from build123d import *

# Parameters (mm, degrees)
F1_DEPTH = 50
F3_D     = 3.3


with BuildPart() as f1:
    # F0 (on Front) → F1 (new body)
    with BuildSketch(Plane.XZ):
        with BuildLine():
            ThreePointArc((-2.9195071176, 0.3029216067), (-2.5916918532, 0.0788381268), (-2.2025121988, 0))
            Line((-2.2025121988, 0), (2.2025121988, 0))
            ThreePointArc((2.2025121988, 0), (2.5916918532, 0.0788381268), (2.9195071176, 0.3029216067))
            Line((2.9195071176, 0.3029216067), (5.1084974594, 2.5544545297))
            ThreePointArc((5.1084974594, 2.5544545297), (5.2132756899, 2.7149096091), (5.25, 2.9029937263))
            Line((5.25, 2.9029937263), (5.25, 3.2))
            ThreePointArc((5.25, 3.2), (5.1035533906, 3.5535533906), (4.75, 3.7))
            Line((4.75, 3.7), (3, 3.7))
            Line((3, 3.7), (3, 7))
            Line((3, 7), (-3, 7))
            Line((-3, 7), (-3, 3.7))
            Line((-3, 3.7), (-4.75, 3.7))
            ThreePointArc((-4.75, 3.7), (-5.1035533906, 3.5535533906), (-5.25, 3.2))
            Line((-5.25, 3.2), (-5.25, 2.9029937263))
            ThreePointArc((-5.25, 2.9029937263), (-5.2132756899, 2.7149096091), (-5.1084974594, 2.5544545297))
            Line((-5.1084974594, 2.5544545297), (-2.9195071176, 0.3029216067))
        make_face()
    extrude(amount=F1_DEPTH)

    # F3 (through all)
    with Locations(Plane.XY.offset(7)):
        with Locations((0, -42.5), (0, -7.5)):
            Hole(F3_D / 2)


solid = f1.part
Can you work these out from the model? Positions are in its coordinate system, mm. A direction names the side the tool comes from. Coordinates: 2 decimals unless noted, no trailing zeros. Order: outer loops, then holes, each group sorted by start corner. A loop starts at its lowest first (then second) coordinate and runs counter-clockwise, first axis right, second up. Notation, with made-up numbers: (52.25, 87) - (72.25, 87) arc R19 cw to (72.25, 123) - close; hole circle Ø9 at (-17.5, 18). An arc over 180 degrees is marked (long way). Answer as a JSON object with one key per item and string values. Group by question number.
Q1. Imagine slicing it at C-C (z = 5.5). Please give me the cut outline in (x, y).
Q2. Imagine slicing it at B-B (x = 0). Please give me the cut outline in (y, z).
Q3. We'd pull the mould along X, two halves only. Please class faces 1 (the face through (3, -25, 5)), 2 (the face through (1.31, -8.5, 3.45)), 3 (the face through (-4.029, -24.65, 1.444)), 4 (the face through (-0.89, -41.11, 3.45)): +X half, -X half, draft (parallel to the pull), parting line (faces both ways), or undercut.
Q4. Imagine slicing it at A-A (y = -7.5). Please give me the cut outline in (x, z).
Q5. Will these pins go through, and if not, where does the flat tip stop? P1, Ø1.6, axis at y = -28, z = 5, coming from the +X side; P2, Ø1.6, axis at y = -28.5, z = 6, coming from the -X side; P3, Ø1.4, axis at x = 4, y = -13.5, coming from the +Z side.
Q6. On a 3-axis mill with a long thin cutter (end or side, diameter ignored), from which of +Z, -Z, +X, -X, +Y, -Y can I reach the whole of each face in a straight line? I mean faces 5 (the face through (-3, -25, 5)), 6 (the face through (0, -25, 0)), 7 (the face through (4, -25, 3.7)). Say none if no direction works.
Q7. Imagine slicing it at D-D (y = -25). Please give me the cut outline in (x, z).
Q8. I need wall thicknesses on line 1 (Y direction, x = 0, z = 4.5); line 2 (X direction, y = -4.5, z = 6.5); line 3 (Y direction, x = 1.5, z = 2.75). Which ranges of each line are inside material? Lowest first, please. Write a range as from..to.
Determined:
{
 "1": {"outline": "(-3, -50) - (3, -50) - (3, 0) - (-3, 0) - close; hole circle Ø3.3 at (0, -42.5); hole circle Ø3.3 at (0, -7.5)"},
 "2": {"outline": "(-50, 0) - (-44.15, 0) - (-44.15, 7) - (-50, 7) - close; (-40.85, 0) - (-9.15, 0) - (-9.15, 7) - (-40.85, 7) - close; (-5.85, 0) - (0, 0) - (0, 7) - (-5.85, 7) - close"},
 "3": {"face 1": "+X half", "face 2": "undercut", "face 3": "-X half", "face 4": "undercut"},
 "4": {"outline": "(-5.25, 2.9) arc R0.5 ccw to (-5.11, 2.55) - (-2.92, 0.3) arc R1 ccw to (-2.2, 0) - (-1.65, 0) - (-1.65, 7) - (-3, 7) - (-3, 3.7) - (-4.75, 3.7) arc R0.5 ccw to (-5.25, 3.2) - close; (1.65, 0) - (2.2, 0) arc R1 ccw to (2.92, 0.3) - (5.11, 2.55) arc R0.5 ccw to (5.25, 2.9) - (5.25, 3.2) arc R0.5 ccw to (4.75, 3.7) - (3, 3.7) - (3, 7) - (1.65, 7) - close"},
 "5": {"P1": "stops at x = 3", "P2": "stops at x = -3", "P3": "stops at z = 3.7"},
 "6": {"face 5": "+Z, -X, +Y, -Y", "face 6": "-Z, +X, -X, +Y, -Y", "face 7": "+Z, +X, +Y, -Y"},
 "7": {"outline": "(-5.25, 2.9) arc R0.5 ccw to (-5.11, 2.55) - (-2.92, 0.3) arc R1 ccw to (-2.2, 0) - (2.2, 0) arc R1 ccw to (2.92, 0.3) - (5.11, 2.55) arc R0.5 ccw to (5.25, 2.9) - (5.25, 3.2) arc R0.5 ccw to (4.75, 3.7) - (3, 3.7) - (3, 7) - (-3, 7) - (-3, 3.7) - (-4.75, 3.7) arc R0.5 ccw to (-5.25, 3.2) - close"},
 "8": {"line 1": "y = -50..-44.15, -40.85..-9.15, -5.85..0", "line 2": "x = -3..3", "line 3": "y = -50..-43.19, -41.81..-8.19, -6.81..0"}
}
